Geometry check sheet. Reference: the model listing, model coordinates, mm. A direction names the side the tool comes from. Give positions to 0.01 mm unless a question says otherwise; leave off trailing zeros. Order: outer loops, then holes, each group sorted by start corner. A loop starts at its lowest first (then second) coordinate and runs counter-clockwise, first axis right, second up. Notation, with made-up numbers: M 42,-1.75 L 77,-1.75 A20 ccw 77,24.25 Z; hole C 88.25,-18.75 d6. An arc over 180 degrees is marked long. One line per question, with ' | ' between items. Start each with the question number.
from build123d import *

# Parameters (mm, degrees)
EXTRUDE_START       = -9.1
EXTRUDE_1_DEPTH     = 6
SKETCH_4_R          = 4.1
CUT_EXTRUDE_3_DEPTH = 4
SKETCH_5_R          = 3.5
CUT_EXTRUDE_5_DEPTH = 28.349588662
SKETCH_6_R          = 1.9
CUT_EXTRUDE_6_DEPTH = 10
EXTRUDE_2_DEPTH     = 3.1
FILLET_1_R          = 2


with BuildPart() as part:
    # ｽｹｯﾁ1 → ﾎﾞｽ - 押し出し1 (new body)
    with BuildSketch(Plane.XY.offset(EXTRUDE_START)):
        with BuildLine():
            Line((0.25, 4.993746089), (-19.7, 5.992495307))
            ThreePointArc((-19.7, 5.992495307), (-26, 0), (-19.7, -5.992495307))
            Line((-19.7, -5.992495307), (0.25, -4.993746089))
            ThreePointArc((0.25, -4.993746089), (5, 0), (0.25, 4.993746089))
        make_face()
    extrude_1 = extrude(amount=EXTRUDE_1_DEPTH)

    # ｽｹｯﾁ4 → ｶｯﾄ - 押し出し3 (cut)
    with BuildSketch(Plane.XY.offset(-3.1)):
        with Locations((-20, 0)):
            Circle(SKETCH_4_R)
    cut_extrude_3 = extrude(amount=-CUT_EXTRUDE_3_DEPTH, mode=Mode.SUBTRACT)

    # ｽｹｯﾁ5 → ｶｯﾄ - 押し出し5 (cut, through all)
    with BuildSketch(Plane.XY.offset(-3.1)):
        with Locations((-20, 0)):
            Circle(SKETCH_5_R)
    cut_extrude_5 = extrude(amount=-CUT_EXTRUDE_5_DEPTH, mode=Mode.SUBTRACT)

    # ｽｹｯﾁ6 → ｶｯﾄ - 押し出し6 (cut)
    with BuildSketch(Plane.XY.offset(-3.1)):
        Circle(SKETCH_6_R)
    cut_extrude_6 = extrude(amount=-CUT_EXTRUDE_6_DEPTH, mode=Mode.SUBTRACT)

    # ｽｹｯﾁ7 → ﾎﾞｽ - 押し出し2 (add)
    with BuildSketch(Plane.XY.offset(-3.1)):
        Polygon((-4, 5.206512213), (-12, 5.607013152), (-12, -5.607013152), (-4, -5.206512213), align=None)
    extrude_2 = extrude(amount=EXTRUDE_2_DEPTH)

    # ﾐﾗｰ3: ﾎﾞｽ - 押し出し1, ｶｯﾄ - 押し出し3, ｶｯﾄ - 押し出し5, ｶｯﾄ - 押し出し6, ﾎﾞｽ - 押し出し2 across plane
    add(extrude_1.mirror(Plane.XY))
    add(cut_extrude_3.mirror(Plane.XY), mode=Mode.SUBTRACT)
    add(cut_extrude_5.mirror(Plane.XY), mode=Mode.SUBTRACT)
    add(cut_extrude_6.mirror(Plane.XY), mode=Mode.SUBTRACT)
    add(extrude_2.mirror(Plane.XY))

    # ﾌｨﾚｯﾄ1
    fillet_1_edges = [part.edges().sort_by_distance(p)[0] for p in [
        (-4, 0, -3.1),
        (-12, 0, -3.1),
        (-4, 0, 3.1),
        (-12, 0, 3.1),
    ]]
    fillet(fillet_1_edges, radius=FILLET_1_R)


solid = part.part
Item 1: Cross-section at D-D, the plane x = -13. Record the cut outline in (y, z), plus the area to 3 significant figures.
Item 2: Cross-section at B-B, the plane z = -6.5. Record the cut outline in (x, y), plus the area to 3 significant figures.
Item 3: Set-up check for faces 3 (the cylindrical face through (-24.096, 0.18, -5.072)), 4 (the cylindrical face through (-3.4, 0.07, 2.53)), 5 (the cylindrical face through (-12.6, -0.08, -2.53)): record each of +Z, -Z, +X, -X, +Y, -Y from which the full face is reachable in a straight line by a thin tool's end or side.
Item 4: Material ranges on line 1 along Z through (x, y) = (-23.5, -2.5); line 2 along X through (y, z) = (-1, -6.75); line 3 along Y through (x, z) = (-20, 6.2), recorded low to high.
Item 5: Cross-section at A-A, the plane x = -22. Record the cut outline in (y, z), plus the area to 3 significant figures.
Item 6: Cross-section at C-C, the plane y = 0. State how many separate pieces and enclosed holes the cut face has, plus the area to 3 significant figures.
Item 7: Mould release check, pull along Z, two halves, no side actions. Record for faces 1 (the cylindrical face through (-24.096, 0.18, 5.072)), 2 (the cylindrical face through (5, 0, 6)): released by +Z, released by -Z, zero draft, split by the parting line, or undercut.
Item 8: Depth check by flat-ended pin: pin 1 (2.5 mm diameter, centred on y = 1.5, z = 0.5, fed in from -X); pin 2 (1.5 mm diameter, centred on x = -8, z = 1, fed in from -Y); pin 3 (5 mm diameter, centred on y = -3.5, z = 2.5, fed in from -X). Enter the tip coordinate at first touch or a pass-through.
Outcome:
1) outline: M -5.66,-9.1 L 5.66,-9.1 L 5.66,-2.83 L -5.66,-2.83 Z; M -5.66,2.83 L 5.66,2.83 L 5.66,9.1 L -5.66,9.1 Z | area: 142 mm²
2) outline: M -19.7,-5.99 L 0.25,-4.99 A5 ccw 0.25,4.99 L -19.7,5.99 A6 ccw long Z; hole C -20,0 d8.2; hole C 0,0 d3.8 | area: 252 mm²
3) face 3: none | face 4: +X, +Y, -Y | face 5: -X, +Y, -Y
4) line 1: z = -9.1 to -3.1, 3.1 to 9.1 | line 2: x = -25.92 to -23.98, -16.02 to -1.62, 1.62 to 4.9 | line 3: y = -6 to -4.1, 4.1 to 6
5) outline: M -5.66,-9.1 L -2.87,-9.1 L -2.87,-7.1 L -3.58,-7.1 L -3.58,-3.1 L -5.66,-3.1 Z; M -5.66,3.1 L -3.58,3.1 L -3.58,7.1 L -2.87,7.1 L -2.87,9.1 L -5.66,9.1 Z; M 2.87,-9.1 L 5.66,-9.1 L 5.66,-3.1 L 3.58,-3.1 L 3.58,-7.1 L 2.87,-7.1 Z; M 2.87,7.1 L 3.58,7.1 L 3.58,3.1 L 5.66,3.1 L 5.66,9.1 L 2.87,9.1 Z | area: 55.5 mm²
6) separate pieces: 5 | enclosed holes: 0 | area: 286 mm²
7) face 1: undercut | face 2: zero draft
8) pin 1: stops at x = -12.11 | pin 2: stops at y = -5.44 | pin 3: stops at x = -25.9
